```python
from build123d import *

# Parameters (mm, degrees)
SKETCH1_R           = 5
BASE_EXTRUDE_DEPTH  = 30
BOSS_EXTRUDE2_DEPTH = 7
CHAMFER1_SIZE       = 1.6


with BuildPart() as part:
    # Sketch1 → Base-Extrude (new body)
    with BuildSketch(Plane.XY):
        Circle(SKETCH1_R)
    extrude(amount=BASE_EXTRUDE_DEPTH)

    # Sketch2 → Boss-Extrude2 (add)
    with BuildSketch(Plane(origin=(0, 0, 0), x_dir=(-1, 0, 0), z_dir=(0, 0, -1))):
        Polygon((0, 9.814954576), (-8.5, 4.907477288), (-8.5, -4.907477288), (0, -9.814954576), (8.5, -4.907477288), (8.5, 4.907477288), align=None)
    extrude(amount=BOSS_EXTRUDE2_DEPTH)

    # Chamfer1
    chamfer1_edges = [part.edges().sort_by_distance(p)[0] for p in [
        (-5, 0, 30),
    ]]
    chamfer(chamfer1_edges, length=CHAMFER1_SIZE)


solid = part.part
```
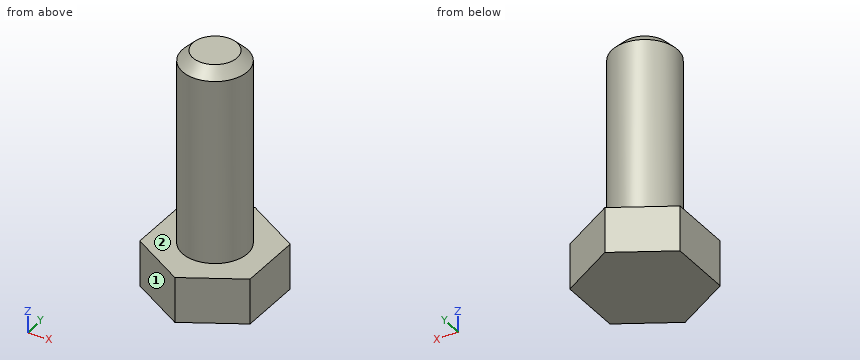
Check sheet for the modelled part. Datum: model origin and axes. Units: mm. Face numbers are marked on the shaded views. A direction names the side the tool comes from. Coordinates: 2 decimals unless noted, no trailing zeros. Loops run counter-clockwise (first coordinate to the right, second up) from the corner with the lowest first, then second, coordinate; pieces in that order, holes last. Notation, with made-up numbers: M 84.25,19 L 134.25,19 A28 cw 134.25,41 Z; hole C 40,-7.75 d3. An arc over 180 degrees is marked long. Answer as a JSON object with one key per item and string values.
1. Sectioned sample at C-C on x = 7.5. Record the cut outline in (y, z), and give its area (3 significant figures).
Outcome:
{"outline": "M -5.48,-7 L 5.48,-7 L 5.48,0 L -5.48,0 Z", "area": "76.8 mm²"}
2. Sectioned sample at B-B on y = 0. Record the cut outline in (x, z).
Outcome:
{"outline": "M -8.5,-7 L 8.5,-7 L 8.5,0 L 5,0 L 5,28.4 L 3.4,30 L -3.4,30 L -5,28.4 L -5,0 L -8.5,0 Z"}
3. Depth check by flat-ended pin: P1, Ø3, axis at y = 6.5, z = -3, coming from the +X side; P2, Ø3, axis at x = -5, z = 7, coming from the -Y side; P3, Ø4, axis at y = -1, z = 15.5, coming from the +X side. Enter the tip coordinate at first touch or a pass-through.
Outcome:
{"P1": "x = 8.34", "P2": "y = -3.57", "P3": "x = 5"}
4. Sectioned sample at D-D on z = 17. Record the cut outline in (x, y).
Outcome:
{"outline": "C 0,0 d10"}
5. Scan lines: L1, parallel to Z at x = -0.25, y = 7; L2, parallel to X at y = -0.25, z = 4; L3, parallel to X at y = 8.5, z = -4.5. Record each from-to range of solid material in increasing order. Write a range as from..to.
Outcome:
{"L1": "-7..0", "L2": "-4.99..4.99", "L3": "-2.28..2.28"}
6. Access from +Z, -Z, +X, -X, +Y, -Y to the whole of each face (thin tool, end or side, straight path). Record for the marked faces 1 and 2.
Outcome:
{"face 1": "+Z, -Z, -X, -Y", "face 2": "+Z"}
7. Sectioned sample at A-A on z = -3. Record the cut outline in (x, y), and give its area (3 significant figures).
Outcome:
{"outline": "M -8.5,-4.91 L 0,-9.81 L 8.5,-4.91 L 8.5,4.91 L 0,9.81 L -8.5,4.91 Z", "area": "250 mm²"}
